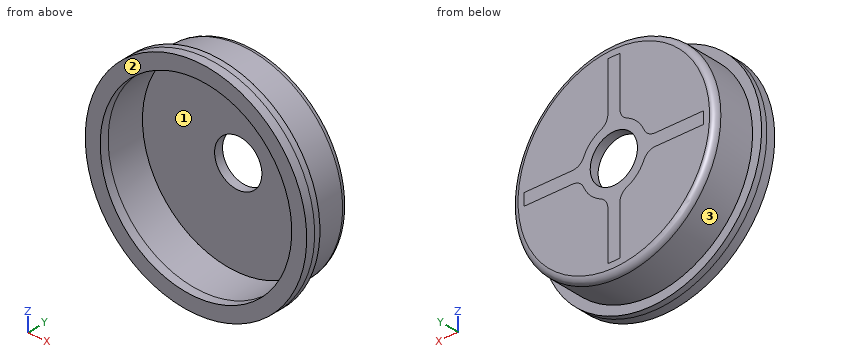
from build123d import *
from build123d.topology import SkipClean

# Parameters (mm, degrees)
SKETCH_1_R          = 18.5
EXTRUDE_1_DEPTH     = 20
SKETCH_2_R          = 16
CUT_EXTRUDE_1_DEPTH = 6.5
SKETCH_3_R          = 3.95
CUT_EXTRUDE_2_DEPTH = 7
SKETCH_4_R          = 3
CUT_EXTRUDE_3_DEPTH = 17
SKETCH_5_R          = 25.146051565
SKETCH_5_R_2        = 17
CUT_EXTRUDE_4_DEPTH = 19
CUT_EXTRUDE_5_DEPTH = 12
FILLET_5_R          = 1
FILLET_7_R          = 2
CUT_EXTRUDE_6_REACH = 34.932
SKETCH_9_R          = 5.408326913
SKETCH_9_R_2        = 4.5
FILLET_8_R          = 0.8
EXTRUDE_START       = 1.5
SKETCH_10_R         = 18.5
SKETCH_10_R_2       = 16
EXTRUDE_2_DEPTH     = 1.5
SKETCH_11_R         = 16
CUT_EXTRUDE_7_DEPTH = 29.783675929


with BuildPart() as part:
    # 草图1 → 凸台-拉伸1 (new body)
    with BuildSketch(Plane(origin=(0, 0, 0), x_dir=(1, 0, 0), z_dir=(0, 1, 0))):
        with Locations(Location((0, 0, 0), (0, 0, 270))):
            Circle(SKETCH_1_R)
    extrude(amount=EXTRUDE_1_DEPTH)

    # 草图2 → 切除-拉伸1 (cut)
    with BuildSketch(Plane.XZ):
        with Locations(Location((0, 0, 0), (0, 0, 270))):
            Circle(SKETCH_2_R)
    extrude(amount=-CUT_EXTRUDE_1_DEPTH, mode=Mode.SUBTRACT)

    # 草图3 → 切除-拉伸2 (cut)
    with BuildSketch(Plane.XZ.offset(-6.5)):
        with Locations(Location((0, 0, 0), (0, 0, 270))):
            Circle(SKETCH_3_R)
    extrude(amount=-CUT_EXTRUDE_2_DEPTH, mode=Mode.SUBTRACT)

    # 草图4 → 切除-拉伸3 (cut)
    with BuildSketch(Plane.XZ.offset(-13.5)):
        with Locations(Location((0, 0, 0), (0, 0, 270))):
            Circle(SKETCH_4_R)
    extrude(amount=-CUT_EXTRUDE_3_DEPTH, mode=Mode.SUBTRACT)

    # 草图5 → 切除-拉伸4 (cut)
    with BuildSketch(Plane(origin=(0, 20, 0), x_dir=(1, 0, 0), z_dir=(0, 1, 0))):
        Circle(SKETCH_5_R)
        with Locations(Location((0, 0, 0), (0, 0, 270))):
            Circle(SKETCH_5_R_2, mode=Mode.SUBTRACT)
    extrude(amount=-CUT_EXTRUDE_4_DEPTH, mode=Mode.SUBTRACT)

    # 草图6 → 切除-拉伸5 (cut)
    with BuildSketch(Plane(origin=(0, 20, 0), x_dir=(1, 0, 0), z_dir=(0, 1, 0))):
        with BuildLine():
            Line((-1, 15.467708298), (-1, 5.408326913))
            ThreePointArc((-1, 5.408326913), (-3.889087297, 3.889087297), (-5.408326913, 1))
            Line((-5.408326913, 1), (-15.467708298, 1))
            ThreePointArc((-15.467708298, 1), (-10.960155108, 10.960155108), (-1, 15.467708298))
        make_face()
        with BuildLine():
            Line((1, 15.467708298), (1, 5.408326913))
            ThreePointArc((1, 5.408326913), (3.889087297, 3.889087297), (5.408326913, 1))
            Line((5.408326913, 1), (15.467708298, 1))
            ThreePointArc((15.467708298, 1), (10.960155108, 10.960155108), (1, 15.467708298))
        make_face()
        with BuildLine():
            Line((-15.467708298, -1), (-5.408326913, -1))
            ThreePointArc((-5.408326913, -1), (-3.889087297, -3.889087297), (-1, -5.408326913))
            Line((-1, -5.408326913), (-1, -15.467708298))
            ThreePointArc((-1, -15.467708298), (-10.960155108, -10.960155108), (-15.467708298, -1))
        make_face()
        with BuildLine():
            Line((1, -5.408326913), (1, -15.467708298))
            ThreePointArc((1, -15.467708298), (10.960155108, -10.960155108), (15.467708298, -1))
            Line((15.467708298, -1), (5.408326913, -1))
            ThreePointArc((5.408326913, -1), (3.889087297, -3.889087297), (1, -5.408326913))
        make_face()
    extrude(amount=-CUT_EXTRUDE_5_DEPTH, mode=Mode.SUBTRACT)

    # 草图8 → 切除-旋转2 (revolve, cut)
    with BuildSketch(Plane.XY, mode=Mode.PRIVATE) as cut_revolve_2_sk:
        Polygon((-19.272016982, 8), (-19.272016982, 20.821833332), (-5.408326913, 20.821833332), (-5.408326913, 16), (-15, 8), (-17, 8), align=None)
    revolve(cut_revolve_2_sk.sketch.rotate(Axis((0, 13.5, 0), (0, -1, 0)), 270), axis=Axis((0, 13.5, 0), (0, -1, 0)), mode=Mode.SUBTRACT)

    # 圆角5
    fillet_5_edges = [part.edges().sort_by_distance(p)[0] for p in [
        (0, 8, -17),
    ]]
    fillet(fillet_5_edges, radius=FILLET_5_R)

    # 圆角7
    fillet_7_edges = [part.edges().sort_by_distance(p)[0] for p in [
        (-1, 11.96176972, 5.408326913),
        (-5.408326913, 11.96176972, 1),
        (-5.408326913, 11.96176972, -1),
        (-1, 11.96176972, -5.408326913),
        (1, 11.96176972, -5.408326913),
        (5.408326913, 11.96176972, -1),
        (5.408326913, 11.96176972, 1),
        (1, 11.96176972, 5.408326913),
    ]]
    fillet(fillet_7_edges, radius=FILLET_7_R)

    # 切除-拉伸6: up to this cone (the profile starts outside it)
    with SkipClean():  # the faces are left unmerged after this step: merging them gives an invalid solid
        cut_extrude_6_end = Plane(origin=(0, 20, 0), z_dir=(0, -1, 0)).offset(-0.510850748) * Cone(1.199e-06, 43.828361396, 36.555341117, align=(Align.CENTER, Align.CENTER, Align.MIN), mode=Mode.PRIVATE)
        # 草图9 → 切除-拉伸6 (cut, up to the surface)
        with BuildSketch(Plane(origin=(0, 20, 0), x_dir=(1, 0, 0), z_dir=(0, 1, 0)), mode=Mode.PRIVATE) as cut_extrude_6_sk1:
            Circle(SKETCH_9_R)
            with Locations(Location((0, 0, 0), (0, 0, 270))):
                Circle(SKETCH_9_R_2, mode=Mode.SUBTRACT)
        cut_extrude_6_tool1 = extrude(cut_extrude_6_sk1.sketch, amount=-CUT_EXTRUDE_6_REACH, mode=Mode.PRIVATE) - cut_extrude_6_end
        add(cut_extrude_6_tool1.solids().sort_by_distance((-5.255356, 20, 0))[0], mode=Mode.SUBTRACT)

    # 圆角8
    fillet_8_edges = [part.edges().sort_by_distance(p)[0] for p in [
        (0, 20, -4.5),
    ]]
    fillet(fillet_8_edges, radius=FILLET_8_R)

    # 草图10 → 凸台-拉伸2 (add)
    with SkipClean():  # the faces are left unmerged after this step: merging them gives an invalid solid
        with BuildSketch(Plane.XZ.offset(EXTRUDE_START)):
            with Locations(Location((0, 0, 0), (0, 0, 270))):
                Circle(SKETCH_10_R)
            with Locations(Location((0, 0, 0), (0, 0, 270))):
                Circle(SKETCH_10_R_2, mode=Mode.SUBTRACT)
        extrude(amount=-EXTRUDE_2_DEPTH)

    # 草图11 → 切除-拉伸7 (cut, through all)
    with BuildSketch(Plane(origin=(0, 8, 0), x_dir=(1, 0, 0), z_dir=(0, 1, 0))):
        with Locations(Location((0, 0, 0), (0, 0, 90))):
            Circle(SKETCH_11_R)
    extrude(amount=CUT_EXTRUDE_7_DEPTH, mode=Mode.SUBTRACT)


solid = part.part
Part model, mm, in its own coordinate system. Face numbers are marked on the shaded views. Give positions to 0.01 mm unless a question says otherwise; leave off trailing zeros. Write each loop counter-clockwise with the first axis right and the second up, starting at its lowest first coordinate (ties: lowest second). Pieces come first, ordered by that corner, then holes.
1) Two-plate mould, pull along X, no slides. Class the marked faces 1, 2 and 3: released by +X, released by -X, zero draft, split by the parting line, or undercut.
Resolved:
face 1: undercut
face 2: zero draft
face 3: split by the parting line
2) Probe L1, parallel to X at y = 1.5, z = 0; L2, parallel to X at y = -1.2, z = 0; L3, parallel to Y at x = 7, z = 5.5. List the from-to ranges inside material, lowest first.
Resolved:
L1: x = -17 to -16, 16 to 17
L2: x = -18.5 to -16, 16 to 18.5
L3: y = 6.5 to 8
3) Cut at A-A on z = 0. Write the cut outline in (x, y).
Resolved:
outline: (-18.5, -1.5) - (-16, -1.5) - (-16, 6.5) - (-3.95, 6.5) - (-3.95, 8) - (-16, 8) arc R1 ccw to (-17, 7) - (-17, 1) - (-18.5, 1) - close; (3.95, 6.5) - (16, 6.5) - (16, -1.5) - (18.5, -1.5) - (18.5, 1) - (17, 1) - (17, 7) arc R1 ccw to (16, 8) - (3.95, 8) - close
4) Pin check, flat tips, straight feed: pin 1 (2 mm diameter, centred on x = -3, y = 2.5, fed in from -Z); pin 2 (12 mm diameter, centred on x = -3, z = 9, fed in from -Y); pin 3 (1 mm diameter, centred on x = 14, y = 6.5, fed in from +Z). Stop position of each tip, or through.
Resolved:
pin 1: stops at z = -16.88
pin 2: stops at y = 6.5
pin 3: stops at z = 10.33
5) Cut at B-B on y = 3. Write the cut outline in (x, z).
Resolved:
outline: circle Ø34 at (0, 0); hole circle Ø32 at (0, 0)
6) Cut at C-C on y = -0.5. Write the cut outline in (x, z), then the cut area to 3 significant figures.
Resolved:
outline: circle Ø37 at (0, 0); hole circle Ø32 at (0, 0)
area: 271 mm2
